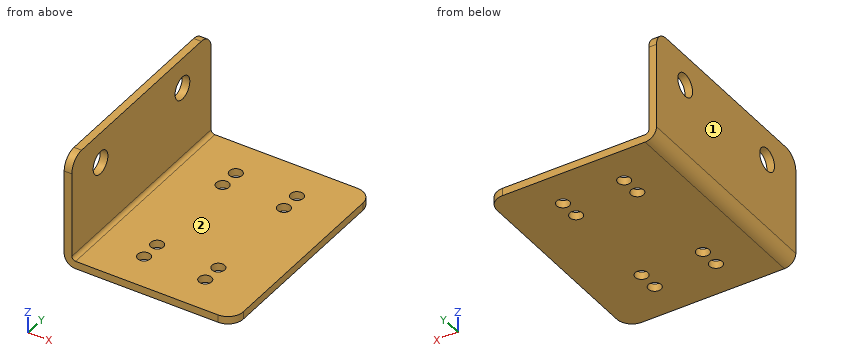
```python
from build123d import *

# Parameters (mm, degrees)
SKETCH_1_W                       = 33.2
SKETCH_1_H                       = 42.5
SM_BASE_FLANGE_1_DEPTH           = 1.5
SM_EDGE_FLANGE_1_STRIP_W         = 7.4732
SM_EDGE_FLANGE_1_STRIP_H         = 1.5
SM_EDGE_FLANGE_1_STRIP_CUT_DEPTH = 42.5
SM_EDGE_FLANGE_1_DEPTH           = 42.5
SKETCH_9_R                       = 1.25
CUT_EXTRUDE_1_DEPTH              = 10
SKETCH_10_R                      = 2.25
CUT_EXTRUDE_2_DEPTH              = 10
FILLET_1_R                       = 3


# Sheet-metal steps are written as plain solids
with BuildPart() as part:
    # Sketch 1 → 基体-法兰1 (new body)
    with BuildSketch(Plane.XY):
        Rectangle(SKETCH_1_W, SKETCH_1_H)
    extrude(amount=-SM_BASE_FLANGE_1_DEPTH)

    # 边线-法兰1 strip (across the edge) → 边线-法兰1 strip cut (cut)
    with BuildSketch(Plane(origin=(-16.6, 21.25, 0), x_dir=(1, 0, 0), z_dir=(0, -1, 0))):
        with Locations((-1.5, -0.75)):
            Rectangle(SM_EDGE_FLANGE_1_STRIP_W, SM_EDGE_FLANGE_1_STRIP_H)
    extrude(amount=SM_EDGE_FLANGE_1_STRIP_CUT_DEPTH, mode=Mode.SUBTRACT)

    # 边线-法兰1 section (across the edge) → 边线-法兰1 (add)
    with BuildSketch(Plane(origin=(-16.6, 21.25, 0), x_dir=(1, 0, 0), z_dir=(0, -1, 0))):
        with BuildLine():
            Line((0, 0.7366), (0, 20.5))
            Line((0, 20.5), (1.5, 20.5))
            Line((1.5, 20.5), (1.5, 0.7366))
            ThreePointArc((1.5, 0.7366), (1.715745145, 0.215745145), (2.2366, 0))
            Line((2.2366, 0), (2.2366, -1.5))
            ThreePointArc((2.2366, -1.5), (0.655084973, -0.844915027), (0, 0.7366))
        make_face()
    extrude(amount=SM_EDGE_FLANGE_1_DEPTH)

    # 草图9 → 切除-拉伸1 (cut)
    with BuildSketch(Plane.XY):
        with Locations((6.4, 14)):
            Circle(SKETCH_9_R)
        with Locations((-5.6, 14)):
            Circle(SKETCH_9_R)
        with Locations((6.4, -10)):
            Circle(SKETCH_9_R)
        with Locations((-5.6, -10)):
            Circle(SKETCH_9_R)
    cut_extrude_1 = extrude(amount=-CUT_EXTRUDE_1_DEPTH, mode=Mode.SUBTRACT)

    # 草图10 → 切除-拉伸2 (cut)
    with BuildSketch(Plane(origin=(-15.1, 0, 0), x_dir=(0, 0, -1), z_dir=(1, 0, 0))):
        with Locations((-14.5, 12.5)):
            Circle(SKETCH_10_R)
        with Locations((-14.5, -12.5)):
            Circle(SKETCH_10_R)
    extrude(amount=-CUT_EXTRUDE_2_DEPTH, mode=Mode.SUBTRACT)

    # 镜向1: 切除-拉伸1 across plane
    add(cut_extrude_1.mirror(Plane.ZX), mode=Mode.SUBTRACT)

    # 圆角1
    fillet_1_edges = [part.edges().sort_by_distance(p)[0] for p in [
        (-15.85, 21.25, 20.5),
        (-15.85, -21.25, 20.5),
        (16.6, 21.25, -0.75),
        (16.6, -21.25, -0.75),
    ]]
    fillet(fillet_1_edges, radius=FILLET_1_R)


solid = part.part
```
For this review, take the finished solid that the model builds, in its own axes (mm). Face numbers are marked on the shaded views. A direction names the side the tool comes from. Give positions to 0.01 mm unless a question says otherwise; leave off trailing zeros. Write each loop counter-clockwise with the first axis right and the second up, starting at its lowest first coordinate (ties: lowest second). Pieces come first, ordered by that corner, then holes. Notation, with made-up numbers: M 35,64.5 L 50,64.5 A26 cw 50,92.5 Z; hole C 35,48.25 d7. An arc over 180 degrees is marked long. Answer as a JSON object with one key per item and string values. Group by question number.
Item 1: Consider section A-A on y = 14. Write out the cut boundary in (x, z).
Item 2: Consider section B-B on z = 16. Write out the cut boundary in (x, y).
Item 3: Consider section D-D on z = 3. Write out the cut boundary in (x, y), plus the area to 4 significant figures.
Item 4: Tool access review of the marked faces 1 and 2: name each direction out of +Z, -Z, +X, -X, +Y, -Y from which nothing blocks a thin tool from reaching the whole face with its end or side.
Item 5: For pin 1 Ø3 at (x, y) = (-5.6, -14) entering from +Z; pin 2 Ø2 at (x, y) = (-5.6, 10) entering from -Z; pin 3 Ø2 at (y, z) = (6.5, 16) entering from +X, all flat-tipped, find the tip position at first contact; note any pin that passes through.
Item 6: Consider section C-C on y = -12. Write out the cut boundary in (x, z).
Item 7: For probe 1 along Y at (x, z) = (-15.45, 14.5); probe 2 along Y at (x, z) = (-5.6, -0.85); probe 3 along X at (y, z) = (10, -0.35), list the stretches that pass through material, from the lowest coordinate up. Write a range as [from, to].
Check result:
{
 "1": {"outline": "M -16.6,0.74 A2.24 ccw -14.36,-1.5 L -6.85,-1.5 L -6.85,0 L -14.36,0 A0.74 cw -15.1,0.74 L -15.1,12.82 L -16.6,12.82 Z; M -16.6,16.18 L -15.1,16.18 L -15.1,20.5 L -16.6,20.5 Z; M -4.35,-1.5 L 5.15,-1.5 L 5.15,0 L -4.35,0 Z; M 7.65,-1.5 L 16.6,-1.5 L 16.6,0 L 7.65,0 Z"},
 "2": {"outline": "M -16.6,-21.25 L -15.1,-21.25 L -15.1,-14.18 L -16.6,-14.18 Z; M -16.6,-10.82 L -15.1,-10.82 L -15.1,10.82 L -16.6,10.82 Z; M -16.6,14.18 L -15.1,14.18 L -15.1,21.25 L -16.6,21.25 Z"},
 "3": {"outline": "M -16.6,-21.25 L -15.1,-21.25 L -15.1,21.25 L -16.6,21.25 Z", "area": "63.75 mm^2"},
 "4": {"face 1": "+Z, -Z, -X, +Y, -Y", "face 2": "+Z, +X, +Y, -Y"},
 "5": {"pin 1": "stops at z = 0", "pin 2": "passes through", "pin 3": "stops at x = -15.1"},
 "6": {"outline": "M -16.6,0.74 A2.24 ccw -14.36,-1.5 L 16.6,-1.5 L 16.6,0 L -14.36,0 A0.74 cw -15.1,0.74 L -15.1,12.31 L -16.6,12.31 Z; M -16.6,16.69 L -15.1,16.69 L -15.1,20.5 L -16.6,20.5 Z"},
 "7": {"probe 1": "y = [-21.25, -14.75], [-10.25, 10.25], [14.75, 21.25]", "probe 2": "y = [-21.25, -15.25], [-12.75, -11.25], [-8.75, 8.75], [11.25, 12.75], [15.25, 21.25]", "probe 3": "x = [-16.32, -6.85], [-4.35, 5.15], [7.65, 16.6]"}
}
